from build123d import *

# Parameters (mm, degrees)
SKETCH_1_R          = 17.5
EXTRUDE_1_DEPTH     = 30
SKETCH_2_R          = 3
EXTRUDE_2_DEPTH     = 15
FILLET_1_R          = 3
SKETCH_3_R          = 1.5
CUT_EXTRUDE_1_DEPTH = 10


with BuildPart() as part:
    # 草图1 → 凸台-拉伸1 (new body)
    with BuildSketch(Plane(origin=(0, 0, 0), x_dir=(1, 0, 0), z_dir=(0, 1, 0))):
        with Locations(Location((0, 0, 0), (0, 0, 270))):
            Circle(SKETCH_1_R)
    extrude(amount=EXTRUDE_1_DEPTH)

    # 草图2 → 凸台-拉伸2 (add)
    with BuildSketch(Plane(origin=(0, 0, 0), x_dir=(-1, 0, 0), z_dir=(0, -1, 0))):
        with Locations(Location((0, 0, 0), (0, 0, 90))):
            Circle(SKETCH_2_R)
    extrude(amount=EXTRUDE_2_DEPTH)

    # 圆角1
    fillet_1_edges = [part.edges().sort_by_distance(p)[0] for p in [
        (0, 0, -17.5),
        (0, 30, -17.5),
    ]]
    fillet(fillet_1_edges, radius=FILLET_1_R)

    # 草图3 → 切除-拉伸1 (cut)
    with BuildSketch(Plane(origin=(929.367009244, -2, 420.329827188), x_dir=(-0.9109625982496437, 0, -0.41248896299205207), z_dir=(0, -1, 0))):
        with Locations(Location((1012, -0.448882386, 0), (0, 0, 65.638716244))):
            Circle(SKETCH_3_R)
        with Locations(Location((1020, 7.551117614, 0), (0, 0, 65.638716244))):
            Circle(SKETCH_3_R)
        with Locations(Location((1028, -0.448882386, 0), (0, 0, 65.638716244))):
            Circle(SKETCH_3_R)
        with Locations(Location((1020, -8.448882386, 0), (0, 0, 65.638716244))):
            Circle(SKETCH_3_R)
    extrude(amount=-CUT_EXTRUDE_1_DEPTH, mode=Mode.SUBTRACT)


solid = part.part
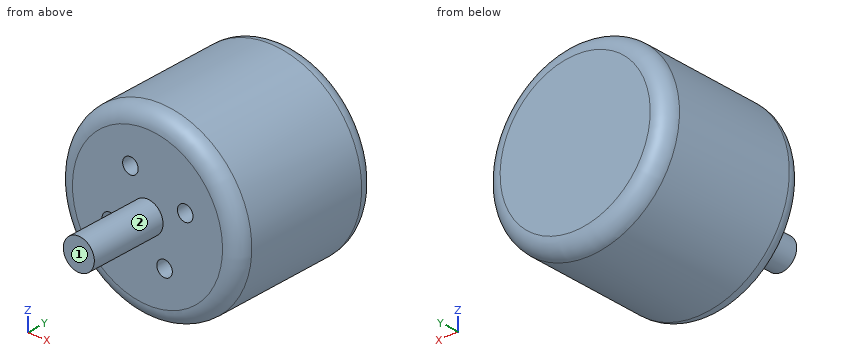
Verification items for the finished model (mm, model axes). Face numbers are marked on the shaded views. A direction names the side the tool comes from. Coordinates: 2 decimals unless noted, no trailing zeros. Write each loop counter-clockwise with the first axis right and the second up, starting at its lowest first coordinate (ties: lowest second). Pieces come first, ordered by that corner, then holes. Notation, with made-up numbers: (39, 46.25) -> (61, 46.25) arc R20 ccw to (61, 85.25) -> close; hole circle Ø7 at (54, -33). An arc over 180 degrees is marked (long way). One line per item, written item: value. Start each with the question number.
Q1. Cross-section at D-D on y = -2. Enter the section's corners in (x, z).
Q2. Thickness scan on L1, parallel to Y at x = 2.5, z = 7.5; L2, parallel to Z at x = 2.5, y = 2.5; L3, parallel to X at y = 4, z = 1. Record the ranges inside material, lowest first. Write a range as from..to.
Q3. Access from +Z, -Z, +X, -X, +Y, -Y to the whole of each face (thin tool, end or side, straight path). Record for the marked faces 1 and 2.
Q4. Cross-section at A-A on x = 0. Enter the section's corners in (y, z), and give its area (3 significant figures).
Q5. Cross-section at B-B on z = 0. Enter the section's corners in (x, y), and give its area (3 significant figures).
Q6. Cross-section at C-C on y = 7. Enter the section's corners in (x, z).
Q7. Go/stop test with flat-tipped pins: P1, Ø12, axis at y = 24.5, z = 0.5, coming from the -X side; P2, Ø3.5, axis at x = -7.5, z = -3, coming from the -Y side; P3, Ø1.5, axis at x = -7, y = 21, coming from the +Z side; P4, Ø1.5, axis at y = 9, z = -11.5, coming from the +X side. Record where each tip stops, or that it passes through.
Checked values:
1. outline: circle Ø6 at (0, 0)
2. L1: y = 0..30
2. L2: z = -17.28..-8.56, -6.02..17.28
2. L3: x = -17.47..17.47
3. face 1: +Z, -Z, +X, -X, -Y
3. face 2: -Y
4. outline: (-15, -3) -> (0, -3) -> (0, -14.5) arc R3 ccw to (3, -17.5) -> (27, -17.5) arc R3 ccw to (30, -14.5) -> (30, 14.5) arc R3 ccw to (27, 17.5) -> (3, 17.5) arc R3 ccw to (0, 14.5) -> (0, 3) -> (-15, 3) -> close
4. area: 1,130 mm²
5. outline: (-17.5, 3) arc R3 ccw to (-14.5, 0) -> (-3, 0) -> (-3, -15) -> (3, -15) -> (3, 0) -> (14.5, 0) arc R3 ccw to (17.5, 3) -> (17.5, 27) arc R3 ccw to (14.5, 30) -> (-14.5, 30) arc R3 ccw to (-17.5, 27) -> close
5. area: 1,130 mm²
6. outline: circle Ø35 at (0, 0); hole circle Ø3 at (-7.29, -3.3); hole circle Ø3 at (-3.3, 7.29); hole circle Ø3 at (3.3, -7.29); hole circle Ø3 at (7.29, 3.3)
7. P1: stops at x = -17.5
7. P2: stops at y = 0
7. P3: stops at z = 16.35
7. P4: stops at x = 13.81
